Geometry check sheet. Reference: the model listing, model coordinates, mm. A direction names the side the tool comes from. Round coordinates to 2 decimals unless told otherwise and drop trailing zeros. Loops run counter-clockwise (first coordinate to the right, second up) from the corner with the lowest first, then second, coordinate; pieces in that order, holes last. Notation, with made-up numbers: M -30.75,57.5 L 19.25,57.5 A16 ccw 19.25,74.5 Z; hole C 58,71.25 d1. An arc over 180 degrees is marked long. Write item = value, one per line.
Autodesk Inventor part; units mm, degrees
ref_plane "YZ Plane" through (0, 0, 0) normal (1, 0, 0) x (0, 1, 0)
ref_plane "XZ Plane" through (0, 0, 0) normal (0, 1, 0) x (-1, 0, 0)
ref_plane "XY Plane" through (0, 0, 0) normal (0, 0, 1) x (1, 0, 0)
sketch "Sketch1" plane through (0, 0, 0) normal (0, 1, 0) x (-1, 0, 0)
  circle A0 centre (0, 0) radius 2.032
  dimension "d0" = 4.064
extrude "Extrusion1" add sketch "Sketch1" along normal blind 13.335
sketch "Sketch2" plane through (0, 13.335, 0) normal (0, 1, 0) x (1, 0, 0)
  circle A0 centre (0, 0) radius 2.032
  line L0 (1.4368, 1.4368) -> (-1.4368, 1.4368)
  line L1 (-1.4368, 1.4368) -> (-1.4368, -1.4368)
  line L2 (-1.4368, -1.4368) -> (1.4368, -1.4368)
  line L3 (1.4368, -1.4368) -> (1.4368, 1.4368)
  line L4 (1.4368, 1.4368) -> (-1.4368, -1.4368) construction
  line L5 (-1.4368, 1.4368) -> (1.4368, -1.4368) construction
extrude "Extrusion2" add sketch "Sketch2" along normal blind 25.4 contours L3 L2 L1 L0
hole "Hole2" at (0, 0, 0) direction (0, 1, 0) diameter 2.54 depth 15.875
properties part number "shaft_adapter"
(1) Material ranges on line 1 along Z through (x, y) = (0, 12.75); line 2 along Z through (x, y) = (-0.4, 20.5), recorded low to high. Write a range as from..to.
Result set:
line_1 = -2.03..-1.27, 1.27..2.03
line_2 = -1.44..1.44
(2) Sectioned sample at B-B on x = 0. Record the cut outline in (y, z) (3 decimals).
Result set:
outline = M 0,-2.032 L 13.335,-2.032 L 13.335,-1.437 L 38.735,-1.437 L 38.735,1.437 L 13.335,1.437 L 13.335,2.032 L 0,2.032 L 0,1.27 L 15.875,1.27 L 15.875,-1.27 L 0,-1.27 Z
(3) Release check for a two-part mould opening along X. For faces 6 (the cylindrical face through (-1.26, 8.05, 0.17)), 7 (the flat face through (0, 38.735, 0)), 8 (the flat face through (-1.437, 26, 0)) record: released by +X, released by -X, zero draft, split by the parting line, or undercut.
Result set:
face_6 = undercut
face_7 = zero draft
face_8 = released by -X
(4) Sectioned sample at C-C on y = 7. Record the cut outline in (x, z).
Result set:
outline = C 0,0 d4.06; hole C 0,0 d2.54
(5) Depth check by flat-ended pin: pin 1 Ø0.8 at (x, z) = (0.5, -0.5) entering from -Y (3 decimals); pin 2 Ø1 at (x, y) = (0.5, 21) entering from +Z; pin 3 Ø0.9 at (x, y) = (0, 28.5) entering from -Z. Enter the tip coordinate at first touch or a pass-through.
Result set:
pin_1 = 15.875
pin_2 = 1.44
pin_3 = -1.44
(6) Tool access check on faces 1 (the flat face through (0, 15.875, 0)), 2 (the cylindrical face through (0.44, 6.574, 1.984)), 3 (the flat face through (0, 26, 1.437)), 4 (the flat face through (0, 26, -1.437)), 5 (the flat face through (1.437, 26, 0)). Record the directions out of +Z, -Z, +X, -X, +Y, -Y that give a thin tool (end or side, any length) a straight path to the whole face; none if there is none.
Result set:
face_1 = -Y
face_2 = +Y, -Y
face_3 = +Z, +X, -X, +Y
face_4 = -Z, +X, -X, +Y
face_5 = +Z, -Z, +X, +Y
(7) Sectioned sample at D-D on y = 35. Record the cut outline in (x, z).
Result set:
outline = M -1.44,-1.44 L 1.44,-1.44 L 1.44,1.44 L -1.44,1.44 Z
(8) Sectioned sample at A-A on z = 0. Record the cut outline in (x, y) (3 decimals), then the cut area to 3 significant figures.
Result set:
outline = M -2.032,0 L -1.27,0 L -1.27,15.875 L 1.27,15.875 L 1.27,0 L 2.032,0 L 2.032,13.335 L 1.437,13.335 L 1.437,38.735 L -1.437,38.735 L -1.437,13.335 L -2.032,13.335 Z
area = 86.9 mm2
